Part model, mm, in its own coordinate system. A direction names the side the tool comes from. Round coordinates to 2 decimals unless told otherwise and drop trailing zeros. Loops run counter-clockwise (first coordinate to the right, second up) from the corner with the lowest first, then second, coordinate; pieces in that order, holes last. Notation, with made-up numbers: M -11.75,48.5 L 10.25,48.5 A35 ccw 10.25,82.5 Z; hole C 47.5,1.5 d9. An arc over 180 degrees is marked long. Write each question's results on one line, items separated by ' | '.
from build123d import *

# Parameters (mm, degrees)
F1_DEPTH       = 450
F3_D           = 13
F3_DEPTH       = 25
F3_CBORE_D     = 22
F3_CBORE_DEPTH = 13
F3_TIP         = 3.9055940237
F5_D           = 13
F5_DEPTH       = 25
F5_CBORE_D     = 22
F5_CBORE_DEPTH = 13
F5_TIP         = 3.9055940237
F7_D           = 8.8
F7_DEPTH       = 25
F7_TIP         = 2.6437867237
F8_D           = 10
F8_DEPTH       = 12
F8_TIP         = 3.0043030951
F9_SIZE2       = 1
F9_SIZE        = 1


with BuildPart() as f1:
    # F0 (on Front) → F1 (new body)
    with BuildSketch(Plane.XZ):
        Polygon((94, 0), (0, 0), (0, 4), (-66, 4), (-66, -19), (94, -19), align=None)
    extrude(amount=-F1_DEPTH)

    # F3
    with Locations(Plane.XY.offset(4)):
        with Locations((-41, 425), (-41, 344), (-41, 104), (-41, 14)):
            CounterBoreHole(F3_D / 2, F3_CBORE_D / 2, F3_CBORE_DEPTH, depth=F3_DEPTH)
            with Locations((0, 0, -(F3_DEPTH + F3_TIP / 2))):  # 118° drill point
                Cone(0, F3_D / 2, F3_TIP, mode=Mode.SUBTRACT)

    # F5
    with Locations(Plane.XY):
        with Locations((69, 425), (69, 344), (69, 104), (69, 14)):
            CounterBoreHole(F5_D / 2, F5_CBORE_D / 2, F5_CBORE_DEPTH, depth=F5_DEPTH)
            with Locations((0, 0, -(F5_DEPTH + F5_TIP / 2))):  # 118° drill point
                Cone(0, F5_D / 2, F5_TIP, mode=Mode.SUBTRACT)

    # F7
    with Locations(Plane.XY):
        with Locations((14, 25), (14, 105), (14, 185), (14, 265), (14, 345), (14, 425)):
            Hole(F7_D / 2, depth=F7_DEPTH)
            with Locations((0, 0, -(F7_DEPTH + F7_TIP / 2))):  # 118° drill point
                Cone(0, F7_D / 2, F7_TIP, mode=Mode.SUBTRACT)

    # F8
    with Locations(Plane.XY):
        with Locations((14, 120), (14, 360)):
            Hole(F8_D / 2, depth=F8_DEPTH)
            with Locations((0, 0, -(F8_DEPTH + F8_TIP / 2))):  # 118° drill point
                Cone(0, F8_D / 2, F8_TIP, mode=Mode.SUBTRACT)

    # F9
    f9_edges = [f1.edges().sort_by_distance(p)[0] for p in [
        (94, 225, 0),
        (-66, 225, 4),
        (94, 225, -19),
        (-66, 225, -19),
    ]]
    chamfer(f9_edges, length=F9_SIZE, length2=F9_SIZE2)


solid = f1.part
Item 1: Band-saw the part on A-A on y = 425. Count the separate pieces of the cut face and the enclosed holes in it, and give its area (3 significant figures).
Filled sheet:
separate pieces: 4 | enclosed holes: 0 | area: 2,350 mm^2
Item 2: Two-plate mould, pull along Y, no slides. Class faces 1 (the cylindrical face through (-36.209, 18.393, -14.07)), 2 (the flat face through (-66, 222, -7)): +Y half, -Y half, draft (parallel to the pull), parting line (faces both ways), or undercut.
Filled sheet:
face 1: undercut | face 2: draft
Item 3: Wall check: L1, parallel to Y at x = -41, z = -13.5; L2, parallel to X at y = 424, z = -5.5; L3, parallel to Z at x = 3.5, y = 155.5. Give the ranges that are in metal, low to high.
Filled sheet:
L1: 0 to 7.5, 20.5 to 97.5, 110.5 to 337.5, 350.5 to 418.5, 431.5 to 450 | L2: -66 to -51.95, -30.05 to 9.72, 18.28 to 58.05, 79.95 to 94 | L3: -19 to 0
Item 4: Which spindle directions (+Z, -Z, +X, -X, +Y, -Y) get a long thin tool onto all of the face, cutting with end or side? Do faces 3 (the cylindrical face through (11.97, 101.096, -9.633)), 4 (the flat face through (47, 222, 0)), 5 (the cylindrical face through (67.568, 114.906, -6.409)). Say none if no direction does.
Filled sheet:
face 3: +Z, -Z | face 4: +Z, +X, +Y, -Y | face 5: +Z
Item 5: Band-saw the part on C-C on y = 265. Give the cut face in (x, z).
Filled sheet:
outline: M -66,-18 L -65,-19 L 9.6,-19 L 9.6,0 L 0,0 L 0,4 L -65,4 L -66,3 Z; M 18.4,-19 L 93,-19 L 94,-18 L 94,-1 L 93,0 L 18.4,0 Z
Item 6: Drop a flat-ended pin along its axis: P1, Ø14, axis at x = 14, y = 265, coming from the +Z side. Give the stop position or say it passes through.
Filled sheet:
P1: z = 0
Item 7: Band-saw the part on D-D on y = 143. Give the cut face in (x, z).
Filled sheet:
outline: M -66,-18 L -65,-19 L 93,-19 L 94,-18 L 94,-1 L 93,0 L 0,0 L 0,4 L -65,4 L -66,3 Z
